```python
from build123d import *

# Parameters (mm, degrees)
SKETCH_1_R      = 13
SKETCH_1_R_2    = 12
EXTRUDE_1_DEPTH = 60
EXTRUDE_START   = -10
SKETCH_2_R      = 16
SKETCH_2_R_2    = 12
EXTRUDE_3_DEPTH = 2
SKETCH_3_R      = 16
SKETCH_3_R_2    = 12
EXTRUDE_4_DEPTH = 2


with BuildPart() as part:
    # Эскиз1 → Бобышка-Вытянуть1 (new body)
    with BuildSketch(Plane(origin=(0, 0, 0), x_dir=(1, 0, 0), z_dir=(0, 1, 0))):
        Circle(SKETCH_1_R)
        Circle(SKETCH_1_R_2, mode=Mode.SUBTRACT)
    extrude(amount=EXTRUDE_1_DEPTH)

    # Эскиз2 → Бобышка-Вытянуть3 (add)
    with BuildSketch(Plane(origin=(0, 60, 0), x_dir=(1, 0, 0), z_dir=(0, 1, 0)).offset(EXTRUDE_START)):
        Circle(SKETCH_2_R)
        Circle(SKETCH_2_R_2, mode=Mode.SUBTRACT)
    extrude(amount=-EXTRUDE_3_DEPTH)

    # Эскиз3 → Бобышка-Вытянуть4 (add)
    with BuildSketch(Plane.XZ.offset(EXTRUDE_START)):
        Circle(SKETCH_3_R)
        Circle(SKETCH_3_R_2, mode=Mode.SUBTRACT)
    extrude(amount=-EXTRUDE_4_DEPTH)


solid = part.part
```
CAD build for the part. Positions are in the model's coordinates, mm. A direction names the side the tool comes from. Give positions to 0.01 mm unless a question says otherwise; leave off trailing zeros. Write each loop counter-clockwise with the first axis right and the second up, starting at its lowest first coordinate (ties: lowest second). Pieces come first, ordered by that corner, then holes. Notation, with made-up numbers: M 21.5,36 L 61.5,36 A13 ccw 61.5,43 Z; hole C -4,-1 d1. An arc over 180 degrees is marked long. Return JSON: item names as keys, results as strings. Group by question number.
(1) Band-saw the part on C-C (y = 56). Give the cut face in (x, z), and give its area (3 significant figures).
(2) 3-axis set-ups, long thin cutter, end or side, ignore diameter. For faces 1 (the face through (-10.316, 4.93, 7.91)), 2 (the face through (-10.316, 29.748, 7.91)), 3 (the face through (-1.3, 50, -13.1)): which of +Z, -Z, +X, -X, +Y, -Y reach the whole face in a straight line?
(3) Mould opens along Z. For faces 4 (the face through (-11.99, 29.58, -0.53)), 5 (the face through (-10.316, 54.93, 7.91)), 6 (the face through (9, 0, 9)) say: pulls with the +Z half, pulls with the -Z half, needs draft (parallel to the pull), parting line crosses it, or undercut.
(4) Band-saw the part on B-B (x = 0). Give the cut face in (y, z), and give its area (3 significant figures).
(5) Band-saw the part on A-A (z = 0). Give the cut face in (x, y).
(6) Drill centre lines: L1, parallel to Z at x = 0, y = 33; L2, parallel to Y at x = 14, z = 7.5; L3, parallel to Z at x = -10, y = 29. Where is each one in solid material? Low to high. Write a range as [from, to].
(7) Flat gauge pins, fed straight in: pin 1 Ø1 at (y, z) = (18.5, 11.5) entering from -X; pin 2 Ø1 at (x, y) = (-5.5, 10.5) entering from -Z; pin 3 Ø1 at (x, y) = (-10.5, 33.5) entering from +Z. Where does each tip first touch, or does it go through?
Entries:
{
 "1": {"outline": "C 0,0 d26; hole C 0,0 d24", "area": "78.5 mm^2"},
 "2": {"face 1": "-Y", "face 2": "none", "face 3": "+Y"},
 "3": {"face 4": "undercut", "face 5": "parting line crosses it", "face 6": "needs draft"},
 "4": {"outline": "M 0,-13 L 10,-13 L 10,-16 L 12,-16 L 12,-13 L 48,-13 L 48,-16 L 50,-16 L 50,-13 L 60,-13 L 60,-12 L 0,-12 Z; M 0,12 L 60,12 L 60,13 L 50,13 L 50,16 L 48,16 L 48,13 L 12,13 L 12,16 L 10,16 L 10,13 L 0,13 Z", "area": "144 mm^2"},
 "5": {"outline": "M -16,10 L -13,10 L -13,0 L -12,0 L -12,60 L -13,60 L -13,50 L -16,50 L -16,48 L -13,48 L -13,12 L -16,12 Z; M 12,0 L 13,0 L 13,10 L 16,10 L 16,12 L 13,12 L 13,48 L 16,48 L 16,50 L 13,50 L 13,60 L 12,60 Z"},
 "6": {"L1": "z = [-13, -12], [12, 13]", "L2": "y = [10, 12], [48, 50]", "L3": "z = [-8.31, -6.63], [6.63, 8.31]"},
 "7": {"pin 1": "stops at x = -6.93", "pin 2": "stops at z = -15.2", "pin 3": "stops at z = 8.31"}
}
